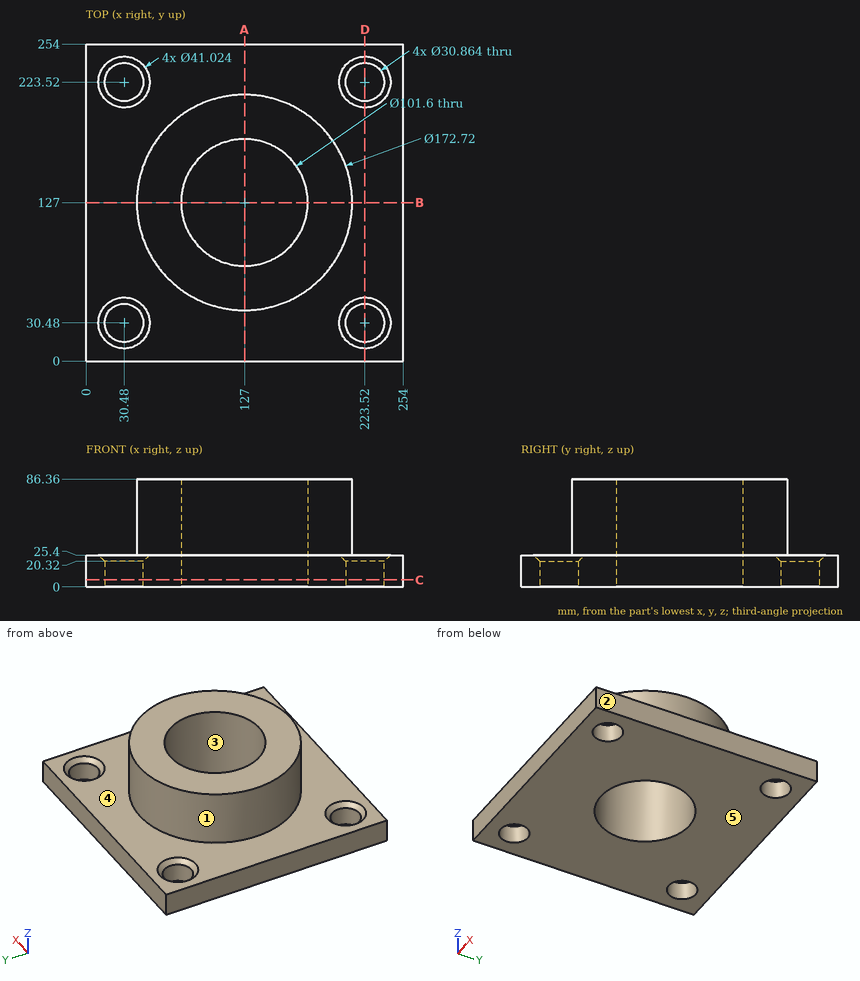
Can you work these out from the drawing? Everything is in mm from the part's minimum corner. A direction names the side the tool comes from. Coordinates: 2 decimals unless noted, no trailing zeros. Loops run counter-clockwise (first coordinate to the right, second up) from the corner with the lowest first, then second, coordinate; pieces in that order, holes last.
1) Imagine slicing it at A-A on x = 127. List the corners of the cut face in (y, z) for me.
2) Imagine slicing it at C-C on z = 5.5. List the corners of the cut face in (x, y) for me.
3) Which directions (+Z, -Z, +X, -X, +Y, -Y) give clear straight access to the entire face, cutting with the end or side of a thin tool? Please do the marked faces 4 and 5.
4) Imagine slicing it at D-D on x = 223.52. State how many separate pieces and enclosed holes the cut face has, plus the area to 3 significant figures.
5) I need wall thicknesses on probe 1 along Y at (x, z) = (30, 10); probe 2 along X at (y, z) = (223.52, 16.25). Which ranges of each line are inside material? Lowest first, please.
6) For pin 1 (2 mm diameter, centred on x = 36, y = 204.5, fed in from +Z); pin 2 (12 mm diameter, centred on y = 82.5, z = 62.5, fed in from -X); pin 3 (5 mm diameter, centred on y = 122, z = 72, fed in from -X), each with a flat end and sliding along its axis, tell me the tip position at first contact or that it passes through.
7) Thinking about a two-plate mould opening in X: for the marked faces 1, 2 and 3, which applies, pulls with the +X half, pulls with the -X half, needs draft (parallel to the pull), parting line crosses it, or undercut?
Completed:
1. outline: (0, 0) - (76.2, 0) - (76.2, 86.36) - (40.64, 86.36) - (40.64, 25.4) - (0, 25.4) - close; (177.8, 0) - (254, 0) - (254, 25.4) - (213.36, 25.4) - (213.36, 86.36) - (177.8, 86.36) - close
2. outline: (0, 0) - (254, 0) - (254, 254) - (0, 254) - close; hole circle Ø30.86 at (30.48, 30.48); hole circle Ø30.86 at (30.48, 223.52); hole circle Ø101.6 at (127, 127); hole circle Ø30.86 at (223.52, 30.48); hole circle Ø30.86 at (223.52, 223.52)
3. face 4: +Z
3. face 5: -Z, +X, -X, +Y, -Y
4. separate pieces: 3
4. enclosed holes: 0
4. area: 4,830 mm2
5. probe 1: y = 0 to 15.06, 45.9 to 208.1, 238.94 to 254
5. probe 2: x = 0 to 15.05, 45.91 to 208.09, 238.95 to 254
6. pin 1: stops at z = 25.4
6. pin 2: stops at x = 49.7
6. pin 3: stops at x = 40.68
7. face 1: parting line crosses it
7. face 2: pulls with the +X half
7. face 3: undercut
